CAD build for the part. Positions are in the model's coordinates, mm. A direction names the side the tool comes from. Give positions to 0.01 mm unless a question says otherwise; leave off trailing zeros. Order: outer loops, then holes, each group sorted by start corner. A loop starts at its lowest first (then second) coordinate and runs counter-clockwise, first axis right, second up. Notation, with made-up numbers: (-19, 8.5) -> (23, 8.5) arc R18 ccw to (23, 18.5) -> close; hole circle Ø9 at (47.5, 9). An arc over 180 degrees is marked (long way). Use one line per item in the form item = value. Start each with the question number.
1) Tool access for faces 1 (the face through (6, 24.218, 5)), 2 (the face through (3, 19.363, 1)), 3 (the face through (-12.96, 20.86, 8.48)): list every direction of +Z, -Z, +X, -X, +Y, -Y with a clear straight run to the whole face (end or side of a thin tool).
2) Probe line 1 (Y direction, x = -2.5, z = 3.5); line 2 (Y direction, x = -18, z = 2); line 3 (X direction, y = 20, z = 2.5). List the from-to ranges inside material, lowest first.
3) Mould opens along X. For faces 4 (the face through (-16, 18, 7)), 5 (the face through (-28.881, 7.467, 5.07)), 6 (the face through (-5.767, 8, 5)) say: pulls with the +X half, pulls with the -X half, needs draft (parallel to the pull), parting line crosses it, or undercut.
4) Cut at B-B, the plane z = 6.5. Give the cut face in (x, y), and give its area (3 significant figures).
5) Cut at A-A, the plane z = 3.5. State how many separate pieces and enclosed holes the cut face has, and give its area (3 significant figures).
6) Drop flat-ended pins along their axis: P1, Ø2, axis at x = -25, y = 15.5, coming from the -Z side; P2, Ø1.2, axis at y = 27.5, z = 3.5, coming from the +X side; P3, Ø2, axis at x = 5, z = 5, coming from the -Y side; P4, Ø2.5, axis at x = 10.23, z = 3.5, coming from the -Y side. Give the stop position or say it passes through.
7) Cut at C-C, the plane x = 2.5. Give the cut face in (y, z).
8) Cut at D-D, the plane y = 10. Give the cut face in (x, z).
from build123d import *

# Parameters (mm, degrees)
ESQUISSE1_R                  = 50
BOSS_EXTRU_1_DEPTH           = 10
ESQUISSE2_R                  = 10
ENL_V_MAT_EXTRU_1_DEPTH      = 7
ESQUISSE4_W                  = 52.254082237
ESQUISSE4_H                  = 3
ENL_V_MAT_EXTRU_2_DEPTH      = 7
ESQUISSE6_W                  = 109.070687356
ESQUISSE6_H                  = 40.053485354
ENL_V_MAT_EXTRU_3_DEPTH      = 10
ESQUISSE8_W                  = 43.455454537
ESQUISSE8_H                  = 73.019440826
ENL_V_MAT_EXTRU_4_DEPTH      = 10
ESQUISSE9_W                  = 83.209839814
ESQUISSE9_H                  = 41.336413251
ENL_V_MAT_EXTRU_5_DEPTH      = 10
ESQUISSE10_W                 = 31.997575123
ESQUISSE10_H                 = 50.623415865
ENL_V_MAT_EXTRU_6_DEPTH      = 10
ESQUISSE11_R                 = 1.5
ENL_V_MAT_EXTRU_7_DEPTH      = 10
CONG_1_R                     = 10
ESQUISSE16_W                 = 20
ESQUISSE16_H                 = 7
ENL_V_MAT_EXTRU_11_DEPTH     = 10
CONG_2_R                     = 3
R_P_TITION_CIRCULAIRE1_COUNT = 4
ESQUISSE17_W                 = 20
ESQUISSE17_H                 = 7.090454939
ENL_V_MAT_EXTRU_12_DEPTH     = 10
CONG_3_R                     = 3
ESQUISSE19_R                 = 2
ENL_V_MAT_EXTRU_13_DEPTH     = 20
ESQUISSE19_3_R               = 2
ENL_V_MAT_EXTRU_14_DEPTH     = 20


with BuildPart() as part:
    # Esquisse1 → Boss.-Extru.1 (new body)
    with BuildSketch(Plane.XY):
        with Locations((-18.393953774, 17.863079719)):
            Circle(ESQUISSE1_R)
    extrude(amount=BOSS_EXTRU_1_DEPTH)

    # Esquisse2 → Enl_v. mat.-Extru.1 (cut)
    with BuildSketch(Plane(origin=(0, 0, 0), x_dir=(-1, 0, 0), z_dir=(0, 0, -1))):
        with Locations((18.393953774, 17.863079719)):
            Circle(ESQUISSE2_R)
    extrude(amount=-ENL_V_MAT_EXTRU_1_DEPTH, mode=Mode.SUBTRACT)

    # Esquisse4 → Enl_v. mat.-Extru.2 (cut)
    with BuildSketch(Plane(origin=(0, 0, 0), x_dir=(-1, 0, 0), z_dir=(0, 0, -1))):
        with Locations((-12.461439017, 17.863079719)):
            Rectangle(ESQUISSE4_W, ESQUISSE4_H)
    extrude(amount=-ENL_V_MAT_EXTRU_2_DEPTH, mode=Mode.SUBTRACT)

    # Esquisse6 → Enl_v. mat.-Extru.3 (cut)
    with BuildSketch(Plane(origin=(0, 0, 0), x_dir=(-1, 0, 0), z_dir=(0, 0, -1))):
        with Locations((22.721030159, 51.335342826)):
            Rectangle(ESQUISSE6_W, ESQUISSE6_H)
    extrude(amount=-ENL_V_MAT_EXTRU_3_DEPTH, mode=Mode.SUBTRACT)

    # Esquisse8 → Enl_v. mat.-Extru.4 (cut)
    with BuildSketch(Plane(origin=(0, 0, 0), x_dir=(-1, 0, 0), z_dir=(0, 0, -1))):
        with Locations((53.615379414, 4.486243449)):
            Rectangle(ESQUISSE8_W, ESQUISSE8_H)
    extrude(amount=-ENL_V_MAT_EXTRU_4_DEPTH, mode=Mode.SUBTRACT)

    # Esquisse9 → Enl_v. mat.-Extru.5 (cut)
    with BuildSketch(Plane(origin=(0, 0, 0), x_dir=(-1, 0, 0), z_dir=(0, 0, -1))):
        with Locations((0.000153838, -16.052922386)):
            Rectangle(ESQUISSE9_W, ESQUISSE9_H)
    extrude(amount=-ENL_V_MAT_EXTRU_5_DEPTH, mode=Mode.SUBTRACT)

    # Esquisse10 → Enl_v. mat.-Extru.6 (cut)
    with BuildSketch(Plane(origin=(0, 0, 0), x_dir=(-1, 0, 0), z_dir=(0, 0, -1))):
        with Locations((-30.231359533, 14.74109753)):
            Rectangle(ESQUISSE10_W, ESQUISSE10_H)
    extrude(amount=-ENL_V_MAT_EXTRU_6_DEPTH, mode=Mode.SUBTRACT)

    # Esquisse11 → Enl_v. mat.-Extru.7 (cut)
    with BuildSketch(Plane(origin=(0, 0, 7), x_dir=(-1, 0, 0), z_dir=(0, 0, -1))):
        with Locations((22.887652145, 23.230264731)):
            Circle(ESQUISSE11_R)
    enl_v_mat_extru_7 = extrude(amount=-ENL_V_MAT_EXTRU_7_DEPTH, mode=Mode.SUBTRACT)

    # Cong_1
    cong_1_edges = [part.edges().sort_by_distance(p)[0] for p in [
        (-31.887652145, 31.308600149, 5),
        (-31.887652145, 4.61528424, 5),
    ]]
    fillet(cong_1_edges, radius=CONG_1_R)

    # Esquisse16 → Enl_v. mat.-Extru.11 (cut)
    with BuildSketch(Plane(origin=(0, 0, 0), x_dir=(-1, 0, 0), z_dir=(0, 0, -1))):
        with Locations((-4.232571971, 8.11528424)):
            Rectangle(ESQUISSE16_W, ESQUISSE16_H)
    extrude(amount=-ENL_V_MAT_EXTRU_11_DEPTH, mode=Mode.SUBTRACT)

    # Cong_2
    cong_2_edges = [part.edges().sort_by_distance(p)[0] for p in [
        (-5.767428029, 11.61528424, 5),
        (-5.767428029, 4.61528424, 5),
    ]]
    fillet(cong_2_edges, radius=CONG_2_R)

    # R_p_tition circulaire1: Enl_v. mat.-Extru.7 ×4 about axis
    r_p_tition_circulaire1_axis = Axis((-18.393953774, 17.863079719, 0), (0, 0, 1))
    for i in range(1, R_P_TITION_CIRCULAIRE1_COUNT):
        add(enl_v_mat_extru_7.rotate(r_p_tition_circulaire1_axis, i * 360 / R_P_TITION_CIRCULAIRE1_COUNT), mode=Mode.SUBTRACT)

    # Esquisse17 → Enl_v. mat.-Extru.12 (cut)
    with BuildSketch(Plane(origin=(0, 0, 0), x_dir=(-1, 0, 0), z_dir=(0, 0, -1))):
        with Locations((-4.232571971, 27.76337268)):
            Rectangle(ESQUISSE17_W, ESQUISSE17_H)
    extrude(amount=-ENL_V_MAT_EXTRU_12_DEPTH, mode=Mode.SUBTRACT)

    # Cong_3
    cong_3_edges = [part.edges().sort_by_distance(p)[0] for p in [
        (-5.767428029, 31.308600149, 5),
        (-5.767428029, 24.21814521, 5),
    ]]
    fillet(cong_3_edges, radius=CONG_3_R)

    # Esquisse19 → Enl_v. mat.-Extru.13 (cut)
    with BuildSketch(Plane.XZ.offset(-11.61528424)):
        with Locations((10.232571971, 3.5)):
            Circle(ESQUISSE19_R)
    extrude(amount=-ENL_V_MAT_EXTRU_13_DEPTH, mode=Mode.SUBTRACT)

    # Esquisse19_3 → Enl_v. mat.-Extru.14 (cut)
    with BuildSketch(Plane.XZ.offset(-11.61528424)):
        with Locations((10.232571971, 3.5)):
            Circle(ESQUISSE19_3_R)
        with Locations((2.232571971, 3.5)):
            Circle(ESQUISSE19_3_R)
    extrude(amount=-ENL_V_MAT_EXTRU_14_DEPTH, mode=Mode.SUBTRACT)


solid = part.part
Result:
q1.face_1 = +Z, -Z, +X, +Y
q1.face_2 = -Z, +X
q1.face_3 = +Z, -Z
q2.line_1 = 11.62 to 16.36, 19.36 to 24.22
q2.line_2 = 4.62 to 7.87, 27.86 to 31.31
q2.line_3 = -31.89 to -28.16, -8.62 to 0.5, 3.96 to 8.5, 11.96 to 14.23
q3.face_4 = undercut
q3.face_5 = pulls with the -X half
q3.face_6 = pulls with the +X half
q4.outline = (-31.89, 14.62) arc R10 ccw to (-21.89, 4.62) -> (-8.77, 4.62) arc R3 ccw to (-5.77, 7.62) -> (-5.77, 8.62) arc R3 cw to (-2.77, 11.62) -> (14.23, 11.62) -> (14.23, 16.36) -> (-8.51, 16.36) arc R10 cw (long way) to (-8.51, 19.36) -> (14.23, 19.36) -> (14.23, 24.22) -> (-2.77, 24.22) arc R3 cw to (-5.77, 27.22) -> (-5.77, 28.31) arc R3 ccw to (-8.77, 31.31) -> (-21.89, 31.31) arc R10 ccw to (-31.89, 21.31) -> close
q4.area = 524 mm²
q5.separate_pieces = 5
q5.enclosed_holes = 0
q5.area = 447 mm²
q6.P1 = 7
q6.P2 = -5.75
q6.P3 = 11.62
q6.P4 = through
q7.outline = (11.62, 0) -> (16.36, 0) -> (16.36, 1.52) -> (11.62, 1.52) -> close; (11.62, 5.48) -> (16.36, 5.48) -> (16.36, 7) -> (19.36, 7) -> (19.36, 5.48) -> (24.22, 5.48) -> (24.22, 10) -> (11.62, 10) -> close; (19.36, 0) -> (24.22, 0) -> (24.22, 1.52) -> (19.36, 1.52) -> close
q8.outline = (-30.76, 0) -> (-24.57, 0) -> (-24.57, 7) -> (-12.22, 7) -> (-12.22, 0) -> (-5.43, 0) -> (-5.43, 10) -> (-30.76, 10) -> close
